For this review, use the dimensioned drawing (mm, ordinates from the lowest corner) and the shaded views. Give positions to 0.01 mm unless a question says otherwise; leave off trailing zeros. Loops run counter-clockwise (first coordinate to the right, second up) from the corner with the lowest first, then second, coordinate; pieces in that order, holes last. Notation, with made-up numbers: (15.5, 57.25) - (54.5, 57.25) arc R11 ccw to (54.5, 65.25) - close; hole circle Ø8 at (-36.5, 86). An arc over 180 degrees is marked (long way). Write each question's results on one line, items separated by ' | '.
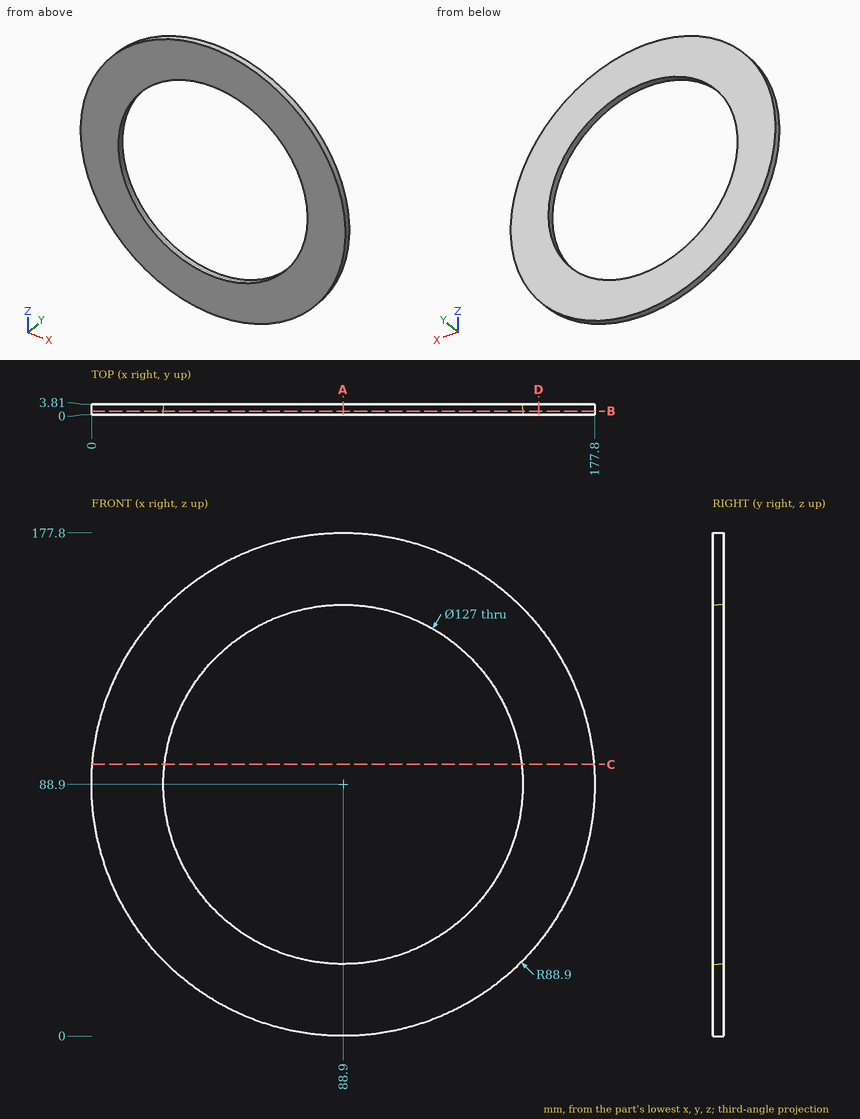
Item 1: We need section B-B on y = 1.3. Give the boundary of the cut face in (x, z) (3 decimals), then the cut area to 3 significant figures.
Output values:
outline: (177.743, 85.725) arc R88.9 ccw to (177.743, 92.075) arc R88.9 ccw (long way) to start; hole circle Ø127 at (88.9, 88.9) | area: 12,200 mm²
Item 2: We need section D-D on x = 158. Give the boundary of the cut face in (y, z).
Output values:
outline: (0, 32.97) - (3.81, 32.97) - (3.81, 144.83) - (0, 144.83) - close
Item 3: Clearance check with flat-ended pins moving along their axes: P1, Ø2, axis at y = 2, z = 56.5, coming from the +X side; P2, Ø1, axis at y = 1.5, z = 81, coming from the +X side; P3, Ø1, axis at y = 1.5, z = 70.5, coming from the +X side. State where each tip first meets the part, or that it passes through.
Output values:
P1: stops at x = 172.07 | P2: stops at x = 177.49 | P3: stops at x = 175.98
Item 4: We need section A-A on x = 88.9. Give the boundary of the cut face in (y, z), then the cut area to 3 significant figures.
Output values:
outline: (0, 0) - (3.81, 0) - (3.81, 25.4) - (0, 25.4) - close; (0, 152.4) - (3.81, 152.4) - (3.81, 177.8) - (0, 177.8) - close | area: 194 mm²
Item 5: We need section C-C on z = 96. Give the boundary of the cut face in (x, y), then the cut area to 3 significant figures.
Output values:
outline: (0.28, 0) - (25.8, 0) - (25.8, 3.81) - (0.28, 3.81) - close; (152, 0) - (177.52, 0) - (177.52, 3.81) - (152, 3.81) - close | area: 194 mm²
Item 6: Wall thickness on probe 1 along Z at (x, y) = (88.9, 1); probe 2 along Z at (x, y) = (31, 3.6): over which ranges is each line inside the solid? List them lowest first.
Output values:
probe 1: z = 0 to 25.4, 152.4 to 177.8 | probe 2: z = 21.44 to 62.83, 114.97 to 156.36
